Autodesk Inventor part; units mm, degrees
ref_plane "YZ Plane" through (0, 0, 0) normal (1, 0, 0) x (0, 1, 0)
ref_plane "XZ Plane" through (0, 0, 0) normal (0, 1, 0) x (-1, 0, 0)
ref_plane "XY Plane" through (0, 0, 0) normal (0, 0, 1) x (1, 0, 0)
sketch "Sketch4" plane through (0, 0, 0) normal (0, 1, 0) x (-1, 0, 0)
  circle A0 centre (0, 0) radius 32
  dimension "d48" = 64
extrude "Extrusion1" add sketch "Sketch4" along normal blind 5
sketch "Sketch5" plane through (0, 5, 0) normal (0, 1, 0) x (1, 0, 0)
  line L0 (-6.5, -32) -> (6.5, -32)
  line L1 (6.5, -32) -> (6.5, -20)
  line L2 (6.5, -20) -> (-6.5, -20)
  line L3 (-6.5, -20) -> (-6.5, -32)
  line L4 (-32, -6.5) -> (-20, -6.5)
  line L5 (-20, -6.5) -> (-20, 6.5)
  line L6 (-20, 6.5) -> (-32, 6.5)
  line L7 (-32, 6.5) -> (-32, -6.5)
  line L8 (-6.5, 20) -> (6.5, 20)
  line L9 (6.5, 20) -> (6.5, 32)
  line L10 (6.5, 32) -> (-6.5, 32)
  line L11 (-6.5, 32) -> (-6.5, 20)
  line L12 (20, -6.5) -> (32, -6.5)
  line L13 (32, -6.5) -> (32, 6.5)
  line L14 (32, 6.5) -> (20, 6.5)
  line L15 (20, 6.5) -> (20, -6.5)
  line L16 (0, 0) -> (-6.9492, 0)
  line L17 (0, 0) -> (0, 8.4834)
  dimension "d51" = 13
  dimension "d52" = 12
  dimension "d53" = 12
  dimension "d54" = 13
  dimension "d57" = 13
  dimension "d58" = 12
  dimension "d59" = 12
  dimension "d60" = 13
  dimension "d61" = 40
  dimension "d62" = 40
extrude "Extrusion2" cut sketch "Sketch5" against normal blind 5
sketch "Sketch6" plane through (0, 5, 0) normal (0, 1, 0) x (1, 0, 0)
  arc A0 (6.5, -31.3329) -> (31.3329, -6.5) centre (0, 0) ccw
  line L0 (31.3329, -6.5) -> (6.5, -6.5)
  line L1 (6.5, -6.5) -> (6.5, -31.3329)
  line L2 (6.5, -31.3329) -> (6.5, -20)
  arc A1 (6.5, -31.3329) -> (31.3329, -6.5) centre (0, 0) ccw
extrude "Extrusion3" add sketch "Sketch6" along normal blind 5
sketch "Sketch7" plane through (0, 5, 0) normal (0, 1, 0) x (1, 0, 0)
  line L0 (-20, 6.5) -> (-20, -6.5)
  line L1 (-20, 6.5) -> (-20, 20)
  line L2 (6.5, 20) -> (-6.5, 20)
  line L3 (-6.5, 20) -> (-20, 20)
  line L4 (-20, 18.5) -> (-13.5, 18.5)
  line L5 (-13.5, 18.5) -> (-13.5, 15.5)
  line L6 (-13.5, 15.5) -> (-20, 15.5)
  line L7 (-20, 15.5) -> (-20, 18.5)
  line L8 (-6.5, 20) -> (-6.5, 31.3329)
  point P0 (0, 0)
  dimension "d69" = 7
  dimension "d70" = 1.5
  dimension "d71" = 6.5
  dimension "d72" = 3
extrude "Extrusion4" add sketch "Sketch7" along normal blind 5
sketch "Sketch8" plane through (0, 0, 0) normal (0, -1, 0) x (1, 0, 0)
  point P0 (0, 0)
sketch "Sketch9" plane through (0, 0, 0) normal (0, -1, 0) x (1, 0, 0)
  line L0 (-31.3329, -6.5) -> (-20, -6.5)
  line L1 (-30.4, -6.5) -> (-21.7, -6.5)
  line L2 (-21.7, -6.5) -> (-21.7, -10.2)
  line L3 (-21.7, -10.2) -> (-30.4, -10.2)
  line L4 (-30.4, -10.2) -> (-30.4, -6.5)
  line L5 (-20, 6.5) -> (-31.3329, 6.5)
  line L6 (-21.7, 6.5) -> (-30.4, 6.5)
  line L7 (-30.4, 6.5) -> (-30.4, 10.2)
  line L8 (-30.4, 10.2) -> (-21.7, 10.2)
  line L9 (-21.7, 10.2) -> (-21.7, 6.5)
  line L10 (6.5, 31.3329) -> (6.5, 20)
  line L11 (6.5, 21.7) -> (10.2, 21.7)
  line L12 (10.2, 21.7) -> (10.2, 30.4)
  line L13 (10.2, 30.4) -> (6.5, 30.4)
  line L14 (6.5, 30.4) -> (6.5, 21.7)
  line L15 (6.5, -31.3329) -> (6.5, -20)
  line L16 (6.5, -21.7) -> (10.2, -21.7)
  line L17 (10.2, -21.7) -> (10.2, -30.4)
  line L18 (10.2, -30.4) -> (6.5, -30.4)
  line L19 (6.5, -30.4) -> (6.5, -21.7)
  line L20 (20, 6.5) -> (31.3329, 6.5)
  line L21 (21.7, 6.5) -> (30.4, 6.5)
  line L22 (30.4, 6.5) -> (30.4, 10.2)
  line L23 (30.4, 10.2) -> (21.7, 10.2)
  line L24 (21.7, 10.2) -> (21.7, 6.5)
  line L25 (21.7, -6.5) -> (30.4, -6.5)
  line L26 (30.4, -6.5) -> (30.4, -10.2)
  line L27 (30.4, -10.2) -> (21.7, -10.2)
  line L28 (21.7, -10.2) -> (21.7, -6.5)
  line L29 (-6.5, -20) -> (-6.5, -31.3329)
  line L30 (-6.5, -30.4) -> (-10.2, -30.4)
  line L31 (-10.2, -30.4) -> (-10.2, -21.7)
  line L32 (-10.2, -21.7) -> (-6.5, -21.7)
  line L33 (-6.5, -21.7) -> (-6.5, -30.4)
  line L34 (-6.5, 31.3329) -> (-6.5, 20)
  line L35 (-10.2, 21.4) -> (-6.5, 21.4)
  line L36 (-6.5, 21.4) -> (-6.5, 30.1)
  line L37 (-6.5, 30.1) -> (-10.2, 30.1)
  line L38 (-10.2, 30.1) -> (-10.2, 21.4)
  line L39 (-6.5, -20) -> (6.5, -20)
  line L40 (20, -6.5) -> (20, 6.5)
  line L41 (6.5, 20) -> (-6.5, 20)
  line L42 (-20, 6.5) -> (-20, -6.5)
  line L43 (-10.2, -29.4) -> (-13.9, -29.4)
  line L44 (-13.9, -29.4) -> (-13.9, -25.1)
  line L45 (-13.9, -25.1) -> (-10.2, -25.1)
  line L46 (-10.2, -25.1) -> (-10.2, -29.4)
  line L47 (-13.9, 20.4) -> (-10.2, 20.4)
  line L48 (-10.2, 20.4) -> (-10.2, 29.1)
  line L49 (-10.2, 29.1) -> (-13.9, 29.1)
  line L50 (-13.9, 29.1) -> (-13.9, 20.4)
  point P0 (0, 0)
  dimension "d75" = 1.7
  dimension "d76" = 8.7
  dimension "d77" = 3.7
  dimension "d78" = 1.7
  dimension "d79" = 8.7
  dimension "d80" = 3.7
  dimension "d81" = 1.7
  dimension "d82" = 3.7
  dimension "d83" = 8.7
  dimension "d84" = 3.7
  dimension "d85" = 8.7
  dimension "d86" = 8.7
  dimension "d87" = 1.7
  dimension "d90" = 1.7
  dimension "d91" = 8.7
  dimension "d96" = 3.7
  dimension "d97" = 4.3
  dimension "d98" = 1
  dimension "d101" = 10.1
  dimension "d102" = 3.7
  dimension "d103" = 8.7
  dimension "d104" = 1
extrude "Extrusion5" add sketch "Sketch9" along normal blind 5
properties part number "Circuit"
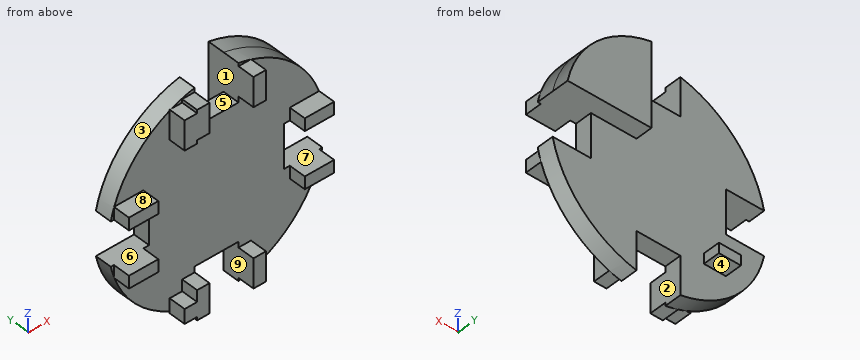
Work out the finished part from the listing and answer in its coordinate system (mm). Face numbers are marked on the shaded views. A direction names the side the tool comes from. Give positions to 0.01 mm unless a question says otherwise; leave off trailing zeros. Loops run counter-clockwise (first coordinate to the right, second up) from the corner with the lowest first, then second, coordinate; pieces in that order, holes last. Notation, with made-up numbers: (82.5, -29) -> (101.5, -29) arc R17 cw to (101.5, -22) -> close; hole circle Ø9 at (-30, 59). An arc over 180 degrees is marked (long way). Write item = value, one per line. Start each with the question number.
(1) Given pin 1 Ø1 at (x, z) = (-7.5, -31) entering from -Y; pin 2 Ø1.8 at (y, z) = (-2.5, -7.5) entering from -X; pin 3 Ø5.5 at (x, y) = (-24.5, -3) entering from +Z, each flat-ended and moving along its own axis, determine where each tip first touches the part or whether it passes through.
(2) Which of the six approach directions +Z, -Z, +X, -X, +Y, -Y give full straight-line access (tool end or side, diameter ignored) to the marked faces 5, 6, 7, 8 and 9?
(3) The mould has two halves that part along X. Classify the marked faces 1, 2, 3 and 4: +X half, -X half, draft (parallel to the pull), parting line (faces both ways), or undercut.
(4) Find section C-C on x = -17. Give the vertices of the cut face in (y, z).
(5) Find section B-B on z = 23. Give the vertices of the cut face in (x, y), and give its area (3 significant figures).
(6) Find the intervals of material crossed by probe 1 along X at (y, z) = (-0.25, 26); probe 2 along Y at (x, z) = (-24, 21); probe 3 along Y at (x, z) = (10.5, 26), in increasing order. Write a range as from..to.
(7) Find section A-A on y = 7.75. Give the vertices of the cut face in (x, z), and give its area (3 significant figures).
(8) Find section D-D on y = -2.75. Give the number of separate pieces and of enclosed holes in the cut face, and give its area (3 significant figures).
From the geometry:
q1.pin_1 = 0
q1.pin_2 = -30.4
q1.pin_3 = 10.2
q2.face_5 = +Z, +Y, -Y
q2.face_6 = -X, +Y, -Y
q2.face_7 = +X, +Y, -Y
q2.face_8 = +Z, +X, -X, -Y
q2.face_9 = -Z, +Y, -Y
q3.face_1 = undercut
q3.face_2 = undercut
q3.face_3 = -X half
q3.face_4 = draft
q4.outline = (0, -27.11) -> (5, -27.11) -> (5, -18.5) -> (10, -18.5) -> (10, -15.5) -> (5, -15.5) -> (5, 27.11) -> (0, 27.11) -> close
q5.outline = (-22.25, 0) -> (-13.9, 0) -> (-13.9, -5) -> (-6.5, -5) -> (-6.5, 5) -> (-22.25, 5) -> close; (6.5, -5) -> (10.2, -5) -> (10.2, 0) -> (22.25, 0) -> (22.25, 10) -> (6.5, 10) -> close
q5.area = 292 mm^2
q6.probe_1 = -13.9..-6.5, 6.5..10.2
q6.probe_2 = 0..5
q6.probe_3 = 0..10
q7.outline = (-20, -18.5) -> (-13.5, -18.5) -> (-13.5, -15.5) -> (-20, -15.5) -> close; (6.5, 6.5) -> (31.33, 6.5) arc R32 ccw to (6.5, 31.33) -> close
q7.area = 453 mm^2
q8.separate_pieces = 8
q8.enclosed_holes = 0
q8.area = 306 mm^2
